Geometry: final body of the model. Coordinates: model frame, mm. A direction names the side the tool comes from. Give positions to 0.01 mm unless a question says otherwise; leave off trailing zeros. Loops run counter-clockwise (first coordinate to the right, second up) from the corner with the lowest first, then second, coordinate; pieces in that order, holes last.
from build123d import *

# Parameters (mm, degrees)
F0_W     = 234.95
F0_H     = 19.05
F1_DEPTH = 19.05
F2_T     = -1.5875
F4_D     = 4.826
F6_D     = 4.826


with BuildPart() as f1:
    # F0 (on Front) → F1 (new body)
    with BuildSketch(Plane.XZ):
        Polygon((-106.4893787249, 190.1872142076), (-125.5393787249, 190.1872142076), (-125.5393787249, -394.0127857924), (-106.4893787249, -394.0127857924), (-106.4893787249, -140.0127857924), (-106.4893787249, -120.9627857924), align=None)
        with Locations((10.9856212751, -130.4877857924)):
            Rectangle(F0_W, F0_H)
        Polygon((128.4606212751, 190.1872142076), (128.4606212751, -120.9627857924), (128.4606212751, -140.0127857924), (128.4606212751, -394.0127857924), (147.5106212751, -394.0127857924), (147.5106212751, 190.1872142076), align=None)
    extrude(amount=F1_DEPTH)

    # F2 (hollow: no face is removed)
    offset(amount=F2_T, kind=Kind.INTERSECTION, mode=Mode.SUBTRACT)

    # F4 (through all)
    with Locations(Plane.YZ.offset(147.5106212751)):
        with Locations((-9.525, -381.3127857924)):
            Hole(F4_D / 2)

    # F6 (through all)
    with Locations(Plane.YZ.offset(147.5106212751)):
        with Locations((-9.525, 177.4872142076)):
            Hole(F6_D / 2)


solid = f1.part
Item 1: Draft query along Y for faces 4 (the face through (10, -19.05, -122)), 5 (the face through (-116, -9, -394.013)), 6 (the face through (-116, -9, -392.425)). Return one class per face: +Y half, -Y half, draft (parallel to the pull), parting line (faces both ways), or undercut.
Values follow:
face 4: -Y half
face 5: draft
face 6: undercut
Item 2: Set-up query: faces 1 (the face through (-106.489, -9, -269)), 2 (the face through (9, -9, -138.425)), 3 (the face through (9, -9, -120.963)). Return all of +Z, -Z, +X, -X, +Y, -Y with unobstructed straight access to the full face (end or side cutting, diameter ignored); none if empty.
Values follow:
face 1: -Z, +Y, -Y
face 2: none
face 3: +Z, +Y, -Y
Item 3: Section query A-A on z = -234. Return loops of the section in (x, y), plus the area to 3 significant figures.
Values follow:
outline: (-125.54, -19.05) - (-106.49, -19.05) - (-106.49, 0) - (-125.54, 0) - close; (128.46, -19.05) - (147.51, -19.05) - (147.51, 0) - (128.46, 0) - close; hole (-123.95, -17.46) - (-108.08, -17.46) - (-108.08, -1.59) - (-123.95, -1.59) - close; hole (130.05, -17.46) - (145.92, -17.46) - (145.92, -1.59) - (130.05, -1.59) - close
area: 222 mm2
Item 4: Ray query, probe 1 along X at (y, z) = (-16.5, -143.5); probe 2 along Z at (x, y) = (-100, -8.25); probe 3 along Y at (x, z) = (-80.5, -128). Return the intervals inside material, ascending.
Values follow:
probe 1: x = -125.54 to -123.95, -108.08 to -106.49, 128.46 to 130.05, 145.92 to 147.51
probe 2: z = -140.01 to -138.43, -122.55 to -120.96
probe 3: y = -19.05 to -17.46, -1.59 to 0
Item 5: Section query B-B on x = -58.5. Return loops of the section in (y, z).
Values follow:
outline: (-19.05, -140.01) - (0, -140.01) - (0, -120.96) - (-19.05, -120.96) - close; hole (-17.46, -138.43) - (-1.59, -138.43) - (-1.59, -122.55) - (-17.46, -122.55) - close
Item 6: Pin query (flat end, axial travel): pin 1 (10 mm diameter, centred on x = 31.5, y = -4, fed in from +Z); pin 2 (3 mm diameter, centred on x = 56.5, y = -2.5, fed in from -Z). Return the tip coordinate at first contact, or that it passes through.
Values follow:
pin 1: stops at z = -120.96
pin 2: stops at z = -140.01
